Build history of the part. All positions in model axes, mm. Face numbers are marked on the shaded views. A direction names the side the tool comes from. Round coordinates to 2 decimals unless told otherwise and drop trailing zeros. Write each loop counter-clockwise with the first axis right and the second up, starting at its lowest first coordinate (ties: lowest second). Pieces come first, ordered by that corner, then holes. Notation, with made-up numbers: (35.5, 63) -> (65.5, 63) arc R27 ccw to (65.5, 92) -> close; hole circle Ø6 at (-9, 3). An arc over 180 degrees is marked (long way). Answer in a Markdown table with one row per item.
```python
from build123d import *

# Parameters (mm, degrees)
SKETCH_1_W                                           = 34
SKETCH_1_H                                           = 41
EXTRUDE_1_DEPTH                                      = 5
FILLET_1_R                                           = 8
SKETCH_2_R                                           = 3
CUT_EXTRUDE_2_DEPTH                                  = 5
SKETCH_3_R                                           = 4
CUT_EXTRUDE_3_DEPTH                                  = 5
SKETCH_4_R                                           = 5
CUT_EXTRUDE_4_DEPTH                                  = 4
HOLE_WIZARD_M2_5_1_D                                 = 2.05
HOLE_WIZARD_M2_5_1_DEPTH                             = 7.35
HOLE_WIZARD_M2_5_1_TIP                               = 0.615882135
CUT_EXTRUDE_5_DEPTH                                  = 10
EXTRUDE1_START                                       = -5
EXTRUDE1_DEPTH                                       = 5
SKETCH_8_R                                           = 1.5
CUT_EXTRUDE_6_DEPTH                                  = 4.5
SKETCH9_R                                            = 0.5
EXTRUDE5_DEPTH                                       = 53.203927134
CUT_EXTRUDE_7_DEPTH                                  = 0.5
CHAMFER_3_SIZE                                       = 0.5
SKETCH2_W                                            = 6
SKETCH2_H                                            = 12
EXTRUDE2_DEPTH                                       = 2
SKETCH7_R                                            = 1.5
EXTRUDE3_DEPTH                                       = 2
EXTRUDE4_DEPTH                                       = 53.249401989
SKETCH10_R                                           = 1.5
EXTRUDE6_DEPTH                                       = 10
CBORE_FOR_M2_5_HEXAGON_SOCKET_HEAD_CAP_S_D           = 2.7
CBORE_FOR_M2_5_HEXAGON_SOCKET_HEAD_CAP_S_CBORE_D     = 5
CBORE_FOR_M2_5_HEXAGON_SOCKET_HEAD_CAP_S_CBORE_DEPTH = 2.5
HOLE_WIZARD_M2_5_1_2_D                               = 2.9
HOLE_WIZARD_M2_5_1_2_CSINK_D                         = 5.5
HOLE_WIZARD_M2_5_1_2_CSINK_ANGLE                     = 90
SKETCH_21_W                                          = 5
SKETCH_21_H                                          = 12
EXTRUDE_1_2_DEPTH                                    = 3
FILLET_2_R                                           = 1
M3X0_5_1_D                                           = 2.5
M3X0_5_1_CSINK_D                                     = 3.05
M3X0_5_1_CSINK_ANGLE                                 = 90


with BuildPart() as part:
    # 草图1 → Extrude 1 (new body)
    with BuildSketch(Plane.XY):
        with Locations((17, 20.5)):
            Rectangle(SKETCH_1_W, SKETCH_1_H)
    extrude(amount=EXTRUDE_1_DEPTH)

    # 圆角1
    fillet_1_edges = [part.edges().sort_by_distance(p)[0] for p in [
        (0, 0, 2.5),
    ]]
    fillet(fillet_1_edges, radius=FILLET_1_R)

    # 草图2 → 拉伸2 (cut)
    with BuildSketch(Plane.XY.offset(5)):
        with Locations((26, 6)):
            Circle(SKETCH_2_R)
    extrude(amount=-CUT_EXTRUDE_2_DEPTH, mode=Mode.SUBTRACT)

    # 草图3 → 拉伸3 (cut)
    with BuildSketch(Plane(origin=(0, 0, 0), x_dir=(-1, 0, 0), z_dir=(0, 0, -1))):
        with Locations((-5.5, 30)):
            Circle(SKETCH_3_R)
    extrude(amount=-CUT_EXTRUDE_3_DEPTH, mode=Mode.SUBTRACT)

    # 草图4 → 拉伸4 (cut)
    with BuildSketch(Plane(origin=(0, 0, 0), x_dir=(-1, 0, 0), z_dir=(0, 0, -1))):
        with Locations((-5.5, 30)):
            Circle(SKETCH_4_R)
    extrude(amount=-CUT_EXTRUDE_4_DEPTH, mode=Mode.SUBTRACT)

    # Hole Wizard M2.5 _1
    with Locations(Plane(origin=(3, 41, 2.5), x_dir=(0, 0, 1), z_dir=(0, 1, 0))):
        with Locations((0, 0), (0, 21)):
            Hole(HOLE_WIZARD_M2_5_1_D / 2, depth=HOLE_WIZARD_M2_5_1_DEPTH)
            with Locations((0, 0, -(HOLE_WIZARD_M2_5_1_DEPTH + HOLE_WIZARD_M2_5_1_TIP / 2))):  # 118° drill point
                Cone(0, HOLE_WIZARD_M2_5_1_D / 2, HOLE_WIZARD_M2_5_1_TIP, mode=Mode.SUBTRACT)

    # 草图7 → 拉伸5 (cut)
    with BuildSketch(Plane(origin=(0, 0, 0), x_dir=(-1, 0, 0), z_dir=(0, 0, -1))):
        with BuildLine():
            Line((-26, 0), (-34, 0))
            Line((-34, 0), (-34, 41))
            Line((-34, 41), (-27.140036221, 41))
            Line((-27.140036221, 41), (-31.941608412, 6.835038606))
            ThreePointArc((-31.941608412, 6.835038606), (-30.528257481, 2.063645826), (-26, 0))
        make_face()
    extrude(amount=-CUT_EXTRUDE_5_DEPTH, mode=Mode.SUBTRACT)

    # Sketch1 → Extrude1 (add)
    with BuildSketch(Plane.XY.offset(5).offset(EXTRUDE1_START)):
        with BuildLine():
            Line((26, 0), (12, 0))
            ThreePointArc((12, 0), (3.514718626, 3.514718626), (0, 12))
            Line((0, 12), (0, 12.980209143))
            Line((0, 12.980209143), (29.441458618, 1.085087734))
            ThreePointArc((29.441458618, 1.085087734), (27.804234797, 0.277698296), (26, 0))
        make_face()
    extrude(amount=EXTRUDE1_DEPTH)

    # 草图8 → 拉伸6 (cut)
    with BuildSketch(Plane.XY.offset(5)):
        with Locations((2.5, 13)):
            Circle(SKETCH_8_R)
    extrude(amount=-CUT_EXTRUDE_6_DEPTH, mode=Mode.SUBTRACT)

    # Sketch9 → Extrude5 (cut, through all)
    with BuildSketch(Plane.XY.offset(0.5)):
        with Locations((1.5, 13)):
            Circle(SKETCH9_R)
    extrude(amount=-EXTRUDE5_DEPTH, mode=Mode.SUBTRACT)

    # 草图9 → 拉伸7 (cut)
    with BuildSketch(Plane.XY.offset(5)):
        with BuildLine():
            Line((0.25, 13), (0.25, 17))
            ThreePointArc((0.25, 17), (2.5, 19.25), (4.75, 17))
            Line((4.75, 17), (4.75, 13))
            ThreePointArc((4.75, 13), (2.5, 10.75), (0.25, 13))
        make_face()
    extrude(amount=-CUT_EXTRUDE_7_DEPTH, mode=Mode.SUBTRACT)

    # 倒角3
    chamfer_3_edges = [part.edges().sort_by_distance(p)[0] for p in [
        (1, 13, 4.5),
    ]]
    chamfer(chamfer_3_edges, length=CHAMFER_3_SIZE)

    # Sketch2 → Extrude2 (cut)
    with BuildSketch(Plane(origin=(0, 0, 0), x_dir=(-1, 0, 0), z_dir=(0, 0, -1))):
        with Locations((-16.5, 27.8)):
            Rectangle(SKETCH2_W, SKETCH2_H)
    extrude(amount=-EXTRUDE2_DEPTH, mode=Mode.SUBTRACT)

    # Sketch7 → Extrude3 (cut)
    with BuildSketch(Plane(origin=(0, 0, 0), x_dir=(-1, 0, 0), z_dir=(0, 0, -1))):
        with Locations((-19.5, 32.3)):
            Circle(SKETCH7_R)
        with Locations((-13.5, 32.3)):
            Circle(SKETCH7_R)
        with Locations((-19.5, 23.3)):
            Circle(SKETCH7_R)
        with Locations((-13.5, 23.3)):
            Circle(SKETCH7_R)
    extrude(amount=-EXTRUDE3_DEPTH, mode=Mode.SUBTRACT)

    # Sketch8 → Extrude4 (cut, through all)
    with BuildSketch(Plane(origin=(0, 0, 0), x_dir=(-1, 0, 0), z_dir=(0, 0, -1))):
        with BuildLine():
            Line((-14, 36), (-14, 41))
            Line((-14, 41), (-19, 41))
            Line((-19, 41), (-19, 36))
            ThreePointArc((-19, 36), (-16.5, 33.5), (-14, 36))
        make_face()
    extrude(amount=-EXTRUDE4_DEPTH, mode=Mode.SUBTRACT)

    # Sketch10 → Extrude6 (cut)
    with BuildSketch(Plane.XY.offset(4.5)):
        with Locations((2.5, 13)):
            Circle(SKETCH10_R)
    extrude(amount=-EXTRUDE6_DEPTH, mode=Mode.SUBTRACT)

    # CBORE for M2.5 Hexagon socket head cap screws1 (through all)
    with Locations(Plane(origin=(4, 6, 0), x_dir=(-1, 0, 0), z_dir=(0, 0, -1))):
        with Locations((0, 0), (-5.5, 5)):
            CounterBoreHole(CBORE_FOR_M2_5_HEXAGON_SOCKET_HEAD_CAP_S_D / 2, CBORE_FOR_M2_5_HEXAGON_SOCKET_HEAD_CAP_S_CBORE_D / 2, CBORE_FOR_M2_5_HEXAGON_SOCKET_HEAD_CAP_S_CBORE_DEPTH)

    # Hole Wizard M2.5 _1 2 (through all)
    with Locations(Plane(origin=(16.5, 30.3, 5), x_dir=(1, 0, 0), z_dir=(0, 0, 1))):
        with Locations((0, 0), (0, -6)):
            CounterSinkHole(HOLE_WIZARD_M2_5_1_2_D / 2, HOLE_WIZARD_M2_5_1_2_CSINK_D / 2, counter_sink_angle=HOLE_WIZARD_M2_5_1_2_CSINK_ANGLE)

    # 草图21 → Extrude 1 2 (add)
    with BuildSketch(Plane.ZY):
        with Locations((2.5, 30)):
            Rectangle(SKETCH_21_W, SKETCH_21_H)
    extrude(amount=EXTRUDE_1_2_DEPTH)

    # 圆角2
    fillet_2_edges = [part.edges().sort_by_distance(p)[0] for p in [
        (0, 24, 2.5),
        (-3, 36, 2.5),
        (-3, 24, 2.5),
        (0, 36, 2.5),
    ]]
    fillet(fillet_2_edges, radius=FILLET_2_R)

    # M3x0.5 螺纹孔1 (through all)
    with Locations(Plane(origin=(7, 38, 5), x_dir=(1, 0, 0), z_dir=(0, 0, 1))):
        with Locations((0, 0)):
            CounterSinkHole(M3X0_5_1_D / 2, M3X0_5_1_CSINK_D / 2, counter_sink_angle=M3X0_5_1_CSINK_ANGLE)


solid = part.part
```
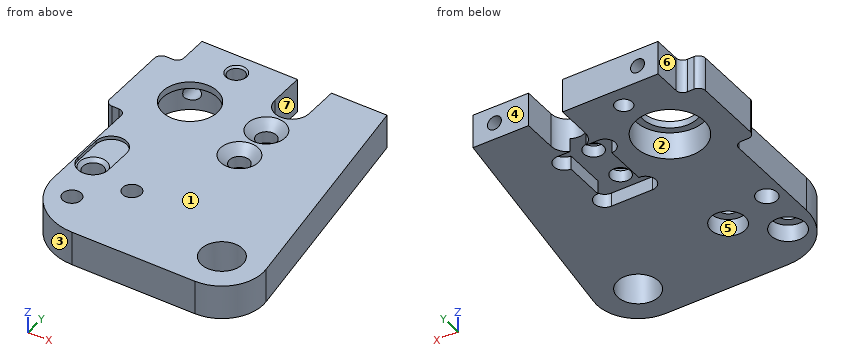
Q1. Drop flat-ended pins along their axis: P1, Ø2.5, axis at x = 4, y = 5.5, coming from the -Z side; P2, Ø3.5, axis at x = 16.5, y = 24.3, coming from the -Z side; P3, Ø1, axis at y = 12.5, z = 1.5, coming from the +X side; P4, Ø1.5, axis at x = 7, y = 38, coming from the +Z side. Give the stop position or say it passes through.
A:
| item | result |
|---|---|
| P1 | z = 2.5 |
| P2 | z = 2 |
| P3 | x = 31.22 |
| P4 | through |
Q2. Which spindle directions (+Z, -Z, +X, -X, +Y, -Y) get a long thin tool onto all of the face, cutting with end or side? Do the marked faces 5, 6 and 7. Say none if no direction does.
A:
| item | result |
|---|---|
| face 5 | -Z |
| face 6 | +Z, -Z, -X, +Y |
| face 7 | +Z, -Z, +Y |
Q3. Saw through at A-A on x = 16.5. Write the cut outline in (y, z), plus the area to 3 significant figures.
A:
| item | result |
|---|---|
| outline | (0, 0) -> (21.8, 0) -> (21.8, 2) -> (22.85, 2) -> (22.85, 3.7) -> (21.55, 5) -> (0, 5) -> close; (25.75, 2) -> (28.85, 2) -> (28.85, 3.7) -> (27.55, 5) -> (27.05, 5) -> (25.75, 3.7) -> close; (31.75, 2) -> (33.5, 2) -> (33.5, 5) -> (33.05, 5) -> (31.75, 3.7) -> close |
| area | 123 mm² |
Q4. Two-plate mould, pull along Y, no slides. Class the marked faces 1, 2, 3 and 4: released by +Y, released by -Y, zero draft, split by the parting line, or undercut.
A:
| item | result |
|---|---|
| face 1 | zero draft |
| face 2 | undercut |
| face 3 | released by -Y |
| face 4 | released by +Y |
Q5. Wall check: line 1 (Y direction, x = 26, z = 4); line 2 (X direction, y = 31, z = 3.6); line 3 (Y direction, x = 7.5, z = 3.9). Give the ranges that are in metal, low to high. Write a range as [from, to].
A:
| item | result |
|---|---|
| line 1 | [0, 3], [9, 41] |
| line 2 | [-3, 0.6], [10.4, 15.23], [17.77, 28.55] |
| line 3 | [0.02, 25.42], [34.58, 36.85], [39.15, 41] |
Q6. Saw through at B-B on z = 0.9. State how many separate pieces and enclosed holes the cut face has, plus the area to 3 significant figures.
A:
| item | result |
|---|---|
| separate pieces | 1 |
| enclosed holes | 6 |
| area | 964 mm² |
Q7. Saw through at C-C on x = 26.5. Write the cut outline in (y, z).
A:
| item | result |
|---|---|
| outline | (0.02, 0) -> (3.04, 0) -> (3.04, 5) -> (0.02, 5) -> close; (8.96, 0) -> (41, 0) -> (41, 5) -> (8.96, 5) -> close |
Q8. Saw through at D-D on y = 18. Write the cut outline in (x, z), plus the area to 3 significant figures.
A:
| item | result |
|---|---|
| outline | (0, 0) -> (30.37, 0) -> (30.37, 5) -> (4.52, 5) -> (4.52, 4.5) -> (0.48, 4.5) -> (0.48, 5) -> (0, 5) -> close |
| area | 150 mm² |
